Autodesk Fusion 360 part; units mm, degrees
sketch "Szkic1" plane through (0, 0, 0) normal (0, 0, 1) x (1, 0, 0)
  line L0 (-13.996, 32.922) -> (69.916, 32.922)
  line L1 (69.916, 32.922) -> (69.916, -68.678)
  line L2 (69.916, -68.678) -> (-13.996, -68.678)
  line L3 (-13.996, -68.678) -> (-13.996, 32.922)
  line L4 (3.025, -2.525) -> (16.025, -2.525)
  line L5 (3.025, -16.525) -> (16.025, -16.525)
  line L6 (2.525, -3.025) -> (2.525, -16.025)
  line L7 (16.525, -3.025) -> (16.525, -16.025)
  arc A0 (3.025, -2.525) -> (2.525, -3.025) centre (3.025, -3.025) ccw
  arc A1 (16.525, -3.025) -> (16.025, -2.525) centre (16.025, -3.025) ccw
  arc A2 (2.525, -16.025) -> (3.025, -16.525) centre (3.025, -16.025) ccw
  arc A3 (16.025, -16.525) -> (16.525, -16.025) centre (16.025, -16.025) ccw
  line L8 (22.075, -2.525) -> (35.075, -2.525)
  line L9 (22.075, -16.525) -> (35.075, -16.525)
  line L10 (21.575, -3.025) -> (21.575, -16.025)
  line L11 (35.575, -3.025) -> (35.575, -16.025)
  arc A4 (22.075, -2.525) -> (21.575, -3.025) centre (22.075, -3.025) ccw
  arc A5 (35.575, -3.025) -> (35.075, -2.525) centre (35.075, -3.025) ccw
  arc A6 (21.575, -16.025) -> (22.075, -16.525) centre (22.075, -16.025) ccw
  arc A7 (35.075, -16.525) -> (35.575, -16.025) centre (35.075, -16.025) ccw
  line L12 (41.125, -2.525) -> (54.125, -2.525)
  line L13 (41.125, -16.525) -> (54.125, -16.525)
  line L14 (40.625, -3.025) -> (40.625, -16.025)
  line L15 (54.625, -3.025) -> (54.625, -16.025)
  arc A8 (41.125, -2.525) -> (40.625, -3.025) centre (41.125, -3.025) ccw
  arc A9 (54.625, -3.025) -> (54.125, -2.525) centre (54.125, -3.025) ccw
  arc A10 (40.625, -16.025) -> (41.125, -16.525) centre (41.125, -16.025) ccw
  arc A11 (54.125, -16.525) -> (54.625, -16.025) centre (54.125, -16.025) ccw
  line L16 (3.025, -21.575) -> (16.025, -21.575)
  line L17 (3.025, -35.575) -> (16.025, -35.575)
  line L18 (2.525, -22.075) -> (2.525, -35.075)
  line L19 (16.525, -22.075) -> (16.525, -35.075)
  arc A12 (3.025, -21.575) -> (2.525, -22.075) centre (3.025, -22.075) ccw
  arc A13 (16.525, -22.075) -> (16.025, -21.575) centre (16.025, -22.075) ccw
  arc A14 (2.525, -35.075) -> (3.025, -35.575) centre (3.025, -35.075) ccw
  arc A15 (16.025, -35.575) -> (16.525, -35.075) centre (16.025, -35.075) ccw
  line L20 (22.075, -21.575) -> (35.075, -21.575)
  line L21 (22.075, -35.575) -> (35.075, -35.575)
  line L22 (21.575, -22.075) -> (21.575, -35.075)
  line L23 (35.575, -22.075) -> (35.575, -35.075)
  arc A16 (22.075, -21.575) -> (21.575, -22.075) centre (22.075, -22.075) ccw
  arc A17 (35.575, -22.075) -> (35.075, -21.575) centre (35.075, -22.075) ccw
  arc A18 (21.575, -35.075) -> (22.075, -35.575) centre (22.075, -35.075) ccw
  arc A19 (35.075, -35.575) -> (35.575, -35.075) centre (35.075, -35.075) ccw
  line L24 (41.125, -21.575) -> (54.125, -21.575)
  line L25 (41.125, -35.575) -> (54.125, -35.575)
  line L26 (40.625, -22.075) -> (40.625, -35.075)
  line L27 (54.625, -22.075) -> (54.625, -35.075)
  arc A20 (41.125, -21.575) -> (40.625, -22.075) centre (41.125, -22.075) ccw
  arc A21 (54.625, -22.075) -> (54.125, -21.575) centre (54.125, -22.075) ccw
  arc A22 (40.625, -35.075) -> (41.125, -35.575) centre (41.125, -35.075) ccw
  arc A23 (54.125, -35.575) -> (54.625, -35.075) centre (54.125, -35.075) ccw
  line L28 (3.025, -40.625) -> (16.025, -40.625)
  line L29 (3.025, -54.625) -> (16.025, -54.625)
  line L30 (2.525, -41.125) -> (2.525, -54.125)
  line L31 (16.525, -41.125) -> (16.525, -54.125)
  arc A24 (3.025, -40.625) -> (2.525, -41.125) centre (3.025, -41.125) ccw
  arc A25 (16.525, -41.125) -> (16.025, -40.625) centre (16.025, -41.125) ccw
  arc A26 (2.525, -54.125) -> (3.025, -54.625) centre (3.025, -54.125) ccw
  arc A27 (16.025, -54.625) -> (16.525, -54.125) centre (16.025, -54.125) ccw
  line L32 (22.075, -40.625) -> (35.075, -40.625)
  line L33 (22.075, -54.625) -> (35.075, -54.625)
  line L34 (21.575, -41.125) -> (21.575, -54.125)
  line L35 (35.575, -41.125) -> (35.575, -54.125)
  arc A28 (22.075, -40.625) -> (21.575, -41.125) centre (22.075, -41.125) ccw
  arc A29 (35.575, -41.125) -> (35.075, -40.625) centre (35.075, -41.125) ccw
  arc A30 (21.575, -54.125) -> (22.075, -54.625) centre (22.075, -54.125) ccw
  arc A31 (35.075, -54.625) -> (35.575, -54.125) centre (35.075, -54.125) ccw
  line L36 (41.125, -40.625) -> (54.125, -40.625)
  line L37 (41.125, -54.625) -> (54.125, -54.625)
  line L38 (40.625, -41.125) -> (40.625, -54.125)
  line L39 (54.625, -41.125) -> (54.625, -54.125)
  arc A32 (41.125, -40.625) -> (40.625, -41.125) centre (41.125, -41.125) ccw
  arc A33 (54.625, -41.125) -> (54.125, -40.625) centre (54.125, -41.125) ccw
  arc A34 (40.625, -54.125) -> (41.125, -54.625) centre (41.125, -54.125) ccw
  arc A35 (54.125, -54.625) -> (54.625, -54.125) centre (54.125, -54.125) ccw
  line L40 (34.533, 21.279) -> (52.033, 21.279)
  line L41 (52.033, 21.279) -> (52.033, 5.879)
  line L42 (52.033, 5.879) -> (34.533, 5.879)
  line L43 (34.533, 5.879) -> (34.533, 21.279)
  dimension "d1" = 16.521
  dimension "d2" = 14.053
  dimension "d3" = 83.912
  dimension "d4" = 101.6
  dimension "d5" = 17.5
  dimension "d6" = 15.4
  dimension "d7" = 8.404
  dimension "d8" = 17.883
extrude "Wyciągnięcie proste1" add sketch "Szkic1" along normal blind 1.5
fillet "Zaokrąglenie1" radius 5 4 edges at (69.916, -68.678, 0.75) (-13.996, -68.678, 0.75) (-13.996, 32.922, 0.75) (69.916, 32.922, 0.75)
Build history of the part. All positions in model axes, mm. Give positions to 0.01 mm unless a question says otherwise; leave off trailing zeros. Order: outer loops, then holes, each group sorted by start corner. A loop starts at its lowest first (then second) coordinate and runs counter-clockwise, first axis right, second up. Notation, with made-up numbers: M 87,76 L 140,76 A15 cw 140,98 Z; hole C 76.5,82 d10. An arc over 180 degrees is marked long. Write item = value, one per line. Start each with the question number.
(1) Slice it at C-C on y = 11.5. Write the cut outline in (x, z).
(2) Slice it at A-A on y = -46. Write the cut outline in (x, z) (3 decimals), plus the area to 3 significant figures.
(3) Slice it at B-B on x = 26. Write the cut outline in (y, z) (3 decimals), plus the area to 3 significant figures.
(4) Slice it at D-D on x = 42.5. Write the cut outline in (y, z) (3 decimals).
(5) Probe L1, parallel to Y at x = 27, z = 0.8 (3 decimals); L2, parallel to Y at x = 49.5, z = 1.3 (3 decimals); L3, parallel to X at y = -7, z = 0.1 (3 decimals). List the from-to ranges inside material, lowest first. Write a range as [from, to].
Responses:
q1.outline = M -14,0 L 34.53,0 L 34.53,1.5 L -14,1.5 Z; M 52.03,0 L 69.92,0 L 69.92,1.5 L 52.03,1.5 Z
q2.outline = M -13.996,0 L 2.525,0 L 2.525,1.5 L -13.996,1.5 Z; M 16.525,0 L 21.575,0 L 21.575,1.5 L 16.525,1.5 Z; M 35.575,0 L 40.625,0 L 40.625,1.5 L 35.575,1.5 Z; M 54.625,0 L 69.916,0 L 69.916,1.5 L 54.625,1.5 Z
q2.area = 62.9 mm2
q3.outline = M -68.678,0 L -54.625,0 L -54.625,1.5 L -68.678,1.5 Z; M -40.625,0 L -35.575,0 L -35.575,1.5 L -40.625,1.5 Z; M -21.575,0 L -16.525,0 L -16.525,1.5 L -21.575,1.5 Z; M -2.525,0 L 32.922,0 L 32.922,1.5 L -2.525,1.5 Z
q3.area = 89.4 mm2
q4.outline = M -68.678,0 L -54.625,0 L -54.625,1.5 L -68.678,1.5 Z; M -40.625,0 L -35.575,0 L -35.575,1.5 L -40.625,1.5 Z; M -21.575,0 L -16.525,0 L -16.525,1.5 L -21.575,1.5 Z; M -2.525,0 L 5.879,0 L 5.879,1.5 L -2.525,1.5 Z; M 21.279,0 L 32.922,0 L 32.922,1.5 L 21.279,1.5 Z
q5.L1 = [-68.678, -54.625], [-40.625, -35.575], [-21.575, -16.525], [-2.525, 32.922]
q5.L2 = [-68.678, -54.625], [-40.625, -35.575], [-21.575, -16.525], [-2.525, 5.879], [21.279, 32.922]
q5.L3 = [-13.996, 2.525], [16.525, 21.575], [35.575, 40.625], [54.625, 69.916]
